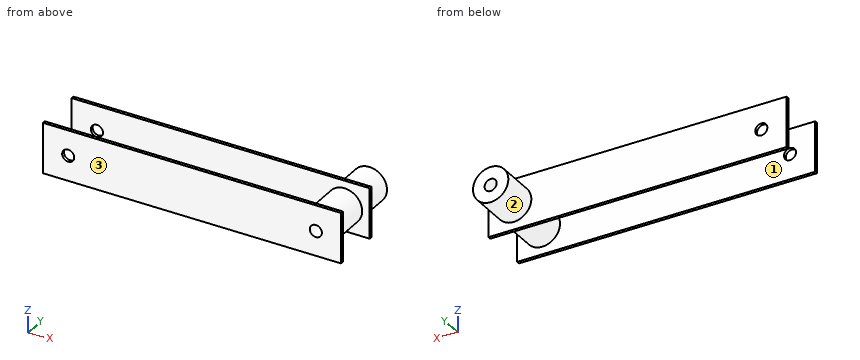
```python
from build123d import *

# Parameters (mm, degrees)
F0_R     = 17.5
F1_DEPTH = 41.5
F2_W     = 295.515
F2_H     = 50
F2_R     = 6
F3_DEPTH = 3
F4_R     = 17.5
F5_DEPTH = 45
F6_W     = 295.515
F6_H     = 50
F6_R     = 6
F7_DEPTH = 3
F8_R     = 6
F9_DEPTH = 89.501


with BuildPart() as f1:
    # F0 (on Front) → F1 (new body)
    with BuildSketch(Plane.XZ):
        Circle(F0_R)
    extrude(amount=F1_DEPTH)

    # F2 (on face) → F3 (join)
    with BuildSketch(Plane.XZ.offset(41.5)):
        with Locations((-122.7575, 0)):
            Rectangle(F2_W, F2_H)
        with Locations((-245.515, 0)):
            Circle(F2_R, mode=Mode.SUBTRACT)
    extrude(amount=-F3_DEPTH)

    # F4 (on face) → F5 (join)
    with BuildSketch(Plane.XZ.offset(41.5)):
        Circle(F4_R)
    extrude(amount=F5_DEPTH)

    # F6 (on face) → F7 (join)
    with BuildSketch(Plane.XZ.offset(86.5)):
        with Locations((-122.7575, 0)):
            Rectangle(F6_W, F6_H)
        with Locations((-245.515, 0)):
            Circle(F6_R, mode=Mode.SUBTRACT)
    extrude(amount=F7_DEPTH)

    # F8 (on Front) → F9 (cut, through all)
    with BuildSketch(Plane.XZ):
        with Locations((0, -0.451715)):
            Circle(F8_R)
    extrude(amount=F9_DEPTH, mode=Mode.SUBTRACT)


solid = f1.part
```
The model under review builds one solid part; all positions refer to its coordinate system, in mm. Face numbers are marked on the shaded views. Give positions to 0.01 mm unless a question says otherwise; leave off trailing zeros. Write each loop counter-clockwise with the first axis right and the second up, starting at its lowest first coordinate (ties: lowest second). Pieces come first, ordered by that corner, then holes. Notation, with made-up numbers: M 13.25,10 L 36.25,10 A24 cw 36.25,23 Z; hole C 8,55.25 d9. An arc over 180 degrees is marked long. Write each question's results on one line, items separated by ' | '. Start each with the question number.
1. For probe 1 along Y at (x, z) = (-177, 11.5); probe 2 along Z at (x, y) = (0, -30.5); probe 3 along X at (y, z) = (-70, -0.5), list the stretches that pass through material, from the lowest coordinate up. Write a range as [from, to].
2. We need section B-B (x = 0). Write out the cut boundary in (y, z).
3. We need section A-A (x = -110). Write out the cut boundary in (y, z), and give its area (3 significant figures).
4. Mouldability with a two-part tool opening along Y and no side actions: class the marked faces 1, 2 and 3 as released by +Y, released by -Y, zero draft, split by the parting line, or undercut.
5. We need section C-C (z = -14.5). Write out the cut boundary in (x, y) (3 decimals), and give its area (3 significant figures).
6. Insertion check: pin 1 Ø15 at (x, z) = (-119.5, 5.5) entering from +Y; pin 2 Ø1 at (y, z) = (-24, 16.5) entering from +X; pin 3 Ø3 at (y, z) = (-54.5, 2) entering from -X. Each pin has a flat end and moves straight along its axis. Give the tip position at first contact, or say it passes through.
Results found:
1) probe 1: y = [-89.5, -86.5], [-41.5, -38.5] | probe 2: z = [-17.5, -6.45], [5.55, 17.5] | probe 3: x = [-17.49, -6], [6, 17.49]
2) outline: M -89.5,-25 L -86.5,-25 L -86.5,-17.5 L -41.5,-17.5 L -41.5,-25 L -38.5,-25 L -38.5,-17.5 L 0,-17.5 L 0,-6.45 L -89.5,-6.45 Z; M -89.5,5.55 L 0,5.55 L 0,17.5 L -38.5,17.5 L -38.5,25 L -41.5,25 L -41.5,17.5 L -86.5,17.5 L -86.5,25 L -89.5,25 Z
3) outline: M -89.5,-25 L -86.5,-25 L -86.5,25 L -89.5,25 Z; M -41.5,-25 L -38.5,-25 L -38.5,25 L -41.5,25 Z | area: 300 mm^2
4) face 1: undercut | face 2: zero draft | face 3: released by -Y
5) outline: M -270.515,-89.5 L 25,-89.5 L 25,-86.5 L 9.798,-86.5 L 9.798,-41.5 L 25,-41.5 L 25,-38.5 L 9.798,-38.5 L 9.798,0 L -9.798,0 L -9.798,-38.5 L -270.515,-38.5 L -270.515,-41.5 L -9.798,-41.5 L -9.798,-86.5 L -270.515,-86.5 Z | area: 3,410 mm^2
6) pin 1: stops at y = -38.5 | pin 2: stops at x = 7.09 | pin 3: stops at x = -17.49
